Geometry: final body of the model. Coordinates: model frame, mm. Face numbers are marked on the shaded views. A direction names the side the tool comes from. Round coordinates to 2 decimals unless told otherwise and drop trailing zeros. Order: outer loops, then holes, each group sorted by start corner. A loop starts at its lowest first (then second) coordinate and runs counter-clockwise, first axis right, second up. Notation, with made-up numbers: (-19, 57) - (-14, 57) arc R27 ccw to (-14, 86) - close; hole circle Ø1 at (20.25, 41.25). An arc over 180 degrees is marked (long way). Put each result on its own line as item: value. Start each with the question number.
(1) Pull-direction query (Z, two-part tool) for the marked faces 1, 2, 3 and 4; classes: released by +Z, released by -Z, zero draft, split by the parting line, or undercut.
(2) Access query for the marked faces 5, 6 and 7. Directions: +Z, -Z, +X, -X, +Y, -Y. A direction counts if a zero-diameter tool reaches every point of the face in a straight line with its end or side. Return the directions, or none.
(3) Section C-C (z = 0.5). Output: boundary loops of the cut face in (x, y), and give its area (3 significant figures).
(4) Pin query (flat end, axial travel): P1, Ø1, axis at x = 17.5, y = 1.5, coming from the -Z side; P2, Ø0.5, axis at x = 19.5, y = 1, coming from the -Z side. Return the tip coordinate at first contact, or that it passes through.
(5) Section A-A (x = 11). Output: boundary loops of the cut face in (y, z).
(6) Section D-D (z = -2.5). Output: boundary loops of the cut face in (x, y), and give its area (3 significant figures).
(7) Material intervals for L1, parallel to Z at x = 16.25, y = 1.3; L2, parallel to Z at x = 17.75, y = 0.7; L3, parallel to Z at x = 19.25, y = 1.8, sorted ascending. Write a range as [from, to].
(8) Section B-B (z = 2). Output: boundary loops of the cut face in (x, y), and give its area (3 significant figures).
from build123d import *

# Parameters (mm, degrees)
BOSS_EXTRUDE1_DEPTH = 2
FILLET1_R           = 0.3


with BuildPart() as part:
    # Sketch1 → Boss-Extrude1 (new body)
    with BuildSketch(Plane(origin=(0, 0, 0), x_dir=(1, 0, 0), z_dir=(0, 1, 0))):
        with BuildLine():
            Line((0, 0), (0, 0.8))
            Line((0, 0.8), (4.8, 1.646369507))
            Line((4.8, 1.646369507), (4.8, 0.8))
            Line((4.8, 0.8), (9.6, 1.646369507))
            Line((9.6, 1.646369507), (9.6, 0.8))
            Line((9.6, 0.8), (14.4, 1.646369507))
            Line((14.4, 1.646369507), (14.4, 0.8))
            Line((14.4, 0.8), (16.4, 0.8))
            Line((16.4, 0.8), (17.54515657, 3.255796188))
            Line((17.54515657, 3.255796188), (18.14515657, 3.255796188))
            Line((18.14515657, 3.255796188), (17, 0.8))
            Line((17, 0.8), (19, 0.8))
            Line((19, 0.8), (19, 2.255796188))
            Line((19, 2.255796188), (20, 2.255796188))
            Line((20, 2.255796188), (20, -2.744203812))
            Line((20, -2.744203812), (19, -2.744203812))
            Line((19, -2.744203812), (19, -1.288407623))
            Line((19, -1.288407623), (17, -1.288407623))
            Line((17, -1.288407623), (18.14515657, -3.744203812))
            Line((18.14515657, -3.744203812), (17.54515657, -3.744203812))
            Line((17.54515657, -3.744203812), (16.4, -1.288407623))
            Line((16.4, -1.288407623), (0, -1.288407623))
            Line((0, -1.288407623), (0, -0.788407623))
            Line((0, -0.788407623), (18.5, -0.788407623))
            ThreePointArc((18.5, -0.788407623), (19, -0.288407623), (18.5, 0.211592377))
            Line((18.5, 0.211592377), (13.8, 0.211592377))
            Line((13.8, 0.211592377), (13.8, 0.952165696))
            Line((13.8, 0.952165696), (9, 0.105796188))
            Line((9, 0.105796188), (9, 0.846369507))
            Line((9, 0.846369507), (4.2, 0))
            Line((4.2, 0), (4.2, 0.740573319))
            Line((4.2, 0.740573319), (0, 0))
        make_face()
    extrude(amount=BOSS_EXTRUDE1_DEPTH)

    # Fillet1
    fillet1_edges = [part.edges().sort_by_distance(p)[0] for p in [
        (0, 1, -0.8),
        (4.8, 1, -0.8),
        (9.6, 1, -0.8),
        (14.4, 1, -0.8),
        (16.4, 1, -0.8),
        (16.4, 1, 1.288407623),
        (13.8, 1, -0.952165696),
        (9, 1, -0.846369507),
        (4.2, 1, -0.740573319),
    ]]
    fillet(fillet1_edges, radius=FILLET1_R)


solid = part.part
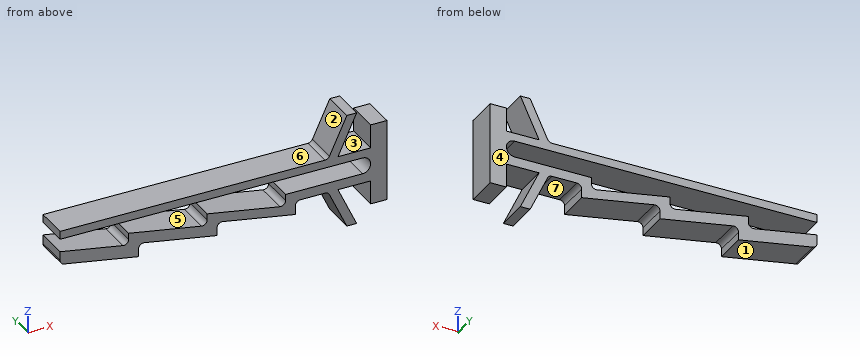
Checks:
1. face 1: released by -Z
1. face 2: released by +Z
1. face 3: undercut
1. face 4: zero draft
2. face 5: +Y, -Y
2. face 6: +Z, -X, +Y, -Y
2. face 7: -Z, +Y, -Y
3. outline: (18.95, 0) - (20, 0) - (20, 2) - (18.95, 2) - close
3. area: 2.09 mm²
4. P1: stops at z = -3.26
4. P2: stops at z = -2.26
5. outline: (0, -1.05) - (2, -1.05) - (2, -0.46) - (0, -0.46) - close; (0, 0.79) - (2, 0.79) - (2, 1.29) - (0, 1.29) - close
6. outline: (17.19, 0) - (17.79, 0) - (17.79, 2) - (17.19, 2) - close
6. area: 1.20 mm²
7. L1: z = [-0.8, -0.21], [0.79, 1.29]
7. L2: z = [-3.26, -2.41], [-0.8, -0.21], [0.79, 1.29], [2.9, 3.74]
7. L3: z = [-2.26, 2.74]
8. outline: (16.73, 0) - (17.33, 0) - (17.33, 2) - (16.73, 2) - close; (19, 0) - (20, 0) - (20, 2) - (19, 2) - close
8. area: 3.20 mm²
